```python
from build123d import *

# Parameters (mm, degrees)
FILLET1_R = 4.7625


with BuildPart() as part:
    # Sketch1 → Revolve1 (revolve)
    with BuildSketch(Plane(origin=(0, 0, 0), x_dir=(0, 0, -1), z_dir=(1, 0, 0))):
        Polygon((-152.4, -7.14375), (152.4, -7.14375), (152.4, 7.14375), (144.4625, 7.14375), (144.4625, 24.60625), (-144.4625, 24.60625), (-144.4625, 7.14375), (-152.4, 7.14375), align=None)
    revolve(axis=Axis((0, -7.14375, 152.4), (0, 0, -1)))

    # Fillet1
    fillet1_edges = [part.edges().sort_by_distance(p)[0] for p in [
        (0, -38.89375, -144.4625),
        (0, -38.89375, 144.4625),
    ]]
    fillet(fillet1_edges, radius=FILLET1_R)


solid = part.part
```
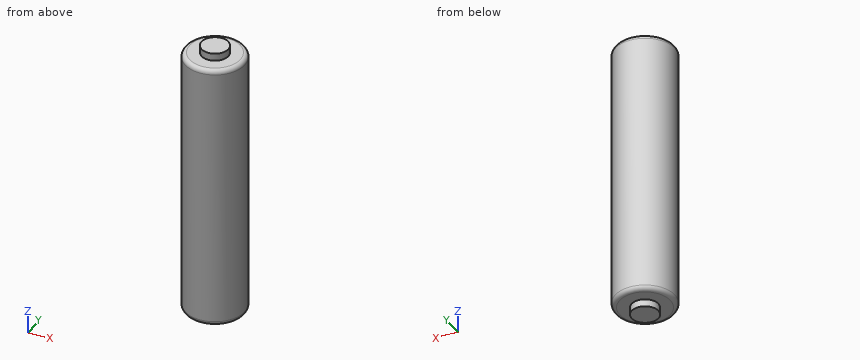
Here's how the part is built. I have some questions about the finished solid (model axes, mm). Give positions to 0.01 mm unless a question says otherwise; leave off trailing zeros. Write each loop counter-clockwise with the first axis right and the second up, starting at its lowest first coordinate (ties: lowest second). Pieces come first, ordered by that corner, then holes. Notation, with made-up numbers: M 89.25,19 L 142.25,19 A13 cw 142.25,37 Z; hole C 45.5,34.5 d2. An arc over 180 degrees is marked long. Put each result on its own line as item: value. Start each with the question number.
Item 1: If we section it at B-B, the plane z = -114: Write out the boundary of the cut face in (x, y), then the cut area to 3 significant figures.
Item 2: Will these pins go through, and if not, where does the flat tip stop? pin 1 (4 mm diameter, centred on x = -20.5, z = 46.5, fed in from -Y); pin 2 (1.5 mm diameter, centred on y = 18, z = 16.5, fed in from -X); pin 3 (10 mm diameter, centred on y = -12, z = -31, fed in from +X).
Item 3: If we section it at A-A, the plane x = 0: Write out the boundary of the cut face in (y, z) (1 decimal).
Item 4: I need wall thicknesses on L1, parallel to Z at x = -17, y = 4; L2, parallel to X at y = -8, z = 114.5; L3, parallel to Y at x = 2, z = 20.5. Which ranges of each line are inside material? Lowest first, please. Write a range as from..to.
Values:
1. outline: C 0,-7.14 d63.5
1. area: 3,170 mm²
2. pin 1: y = -32.95
2. pin 2: x = -20.32
2. pin 3: x = 31.75
3. outline: M -38.9,-139.7 A4.8 ccw -34.1,-144.5 L -21.4,-144.5 L -21.4,-152.4 L 7.1,-152.4 L 7.1,-144.5 L 19.8,-144.5 A4.8 ccw 24.6,-139.7 L 24.6,139.7 A4.8 ccw 19.8,144.5 L 7.1,144.5 L 7.1,152.4 L -21.4,152.4 L -21.4,144.5 L -34.1,144.5 A4.8 ccw -38.9,139.7 Z
4. L1: -144.46..144.46
4. L2: -31.74..31.74
4. L3: -38.83..24.54
